Part model, mm, in its own coordinate system. A direction names the side the tool comes from. Give positions to 0.01 mm unless a question says otherwise; leave off trailing zeros. Order: outer loops, then holes, each group sorted by start corner. A loop starts at its lowest first (then second) coordinate and runs counter-clockwise, first axis right, second up. Notation, with made-up numbers: (23, -36) - (37, -36) arc R20 ccw to (37, -10) - close; hole circle Ø6 at (-17.75, -28.75). An arc over 180 degrees is marked (long way). Use a Markdown table: item, result. Add a question column.
from build123d import *

# Parameters (mm, degrees)
SALIENTE_EXTRUIR2_DEPTH    = 20
CORTAR_EXTRUIR1_DEPTH      = 109.18398602
CORTAR_EXTRUIR1_DEPTH_BACK = 109.18398602
CROQUIS3_R                 = 4
CROQUIS4_R                 = 2
CORTAR_EXTRUIR2_DEPTH      = 109.18398602


with BuildPart() as part:
    # Croquis1 → Saliente-Extruir2 (new body)
    with BuildSketch(Plane.XY):
        with BuildLine():
            Line((-57, 0), (-55.991070717, 0))
            ThreePointArc((-55.991070717, 0), (-55.290305828, -0.286607702), (-54.991230168, -0.982142857))
            ThreePointArc((-54.991230168, -0.982142857), (-41.300644472, -36.32157439), (-8, -54.415071442))
            Line((-8, -54.415071442), (-8, -56.435804238))
            Line((-8, -56.435804238), (-8, -71.312855839))
            Line((-8, -71.312855839), (8, -71.312855839))
            Line((8, -71.312855839), (8, -56.435804238))
            Line((8, -56.435804238), (8, -54.415071442))
            ThreePointArc((8, -54.415071442), (41.300644472, -36.32157439), (54.991230168, -0.982142857))
            ThreePointArc((54.991230168, -0.982142857), (55.290305828, -0.286607702), (55.991070717, 0))
            Line((55.991070717, 0), (57, 0))
            Line((57, 0), (76.5, 0))
            ThreePointArc((76.5, 0), (76.853553391, -0.146446609), (77, -0.5))
            Line((77, -0.5), (77, -1.5))
            ThreePointArc((77, -1.5), (76.853553391, -1.853553391), (76.5, -2))
            Line((76.5, -2), (57.92236183, -2))
            ThreePointArc((57.92236183, -2), (57.233785087, -2.274836523), (56.923700419, -2.948275862))
            ThreePointArc((56.923700419, -2.948275862), (42.736352788, -37.717425023), (10, -56.115951386))
            Line((10, -56.115951386), (10, -73.312855839))
            Line((10, -73.312855839), (-10, -73.312855839))
            Line((-10, -73.312855839), (-10, -56.115951386))
            ThreePointArc((-10, -56.115951386), (-42.736352788, -37.717425023), (-56.923700419, -2.948275862))
            ThreePointArc((-56.923700419, -2.948275862), (-57.233785087, -2.274836523), (-57.92236183, -2))
            Line((-57.92236183, -2), (-76.5, -2))
            ThreePointArc((-76.5, -2), (-76.853553391, -1.853553391), (-77, -1.5))
            Line((-77, -1.5), (-77, -0.5))
            ThreePointArc((-77, -0.5), (-76.853553391, -0.146446609), (-76.5, 0))
            Line((-76.5, 0), (-57, 0))
        make_face()
    extrude(amount=SALIENTE_EXTRUIR2_DEPTH)

    # Croquis3 → Cortar-Extruir1 (cut, two sides: drawn at the far end of the back side and taken through both)
    with BuildSketch(Plane.XZ.offset(73.312855839).offset(-CORTAR_EXTRUIR1_DEPTH_BACK)):
        with Locations(Location((0, 10, 0), (0, 0, 270))):
            Circle(CROQUIS3_R)
    extrude(amount=CORTAR_EXTRUIR1_DEPTH + CORTAR_EXTRUIR1_DEPTH_BACK, mode=Mode.SUBTRACT)

    # Croquis4 → Cortar-Extruir2 (cut, symmetric)
    with BuildSketch(Plane(origin=(0, 0, 0), x_dir=(1, 0, 0), z_dir=(0, 1, 0))):
        with Locations(Location((67, -10, 0), (0, 0, 270))):
            Circle(CROQUIS4_R)
    cortar_extruir2 = extrude(amount=CORTAR_EXTRUIR2_DEPTH, both=True, mode=Mode.SUBTRACT)

    # Simetría1: Cortar-Extruir2 across plane
    add(cortar_extruir2.mirror(Plane(origin=(0, 0, 0), x_dir=(0, 0, 1), z_dir=(1, 0, 0))), mode=Mode.SUBTRACT)


solid = part.part
1. Cut at A-A (x = -67). Write the cut outline in (y, z).
2. Drill centre lines: probe 1 along X at (y, z) = (-1.5, 10); probe 2 along X at (y, z) = (-72.5, 10); probe 3 along Z at (x, y) = (0, -72.65). Where is each one in solid material? Low to high. Write a range as [from, to].
3. Cut at D-D (x = -47). Write the cut outline in (y, z).
4. Mould opens along X. For faces 1 (the face through (43.1, -37.3, 9.9)), 2 (the face through (-66, 0, 12)), 3 (the face through (40.94, -36.73, 9.86)) say: released by +X, released by -X, zero draft, split by the parting line, or undercut.
5. Tool access for faces 4 (the face through (-4, -71.313, 8)), 5 (the face through (-10, -65, 10)), 6 (the face through (69.4, -2, 9.9)), 7 (the face through (69, -1, 10)): list every direction of +Z, -Z, +X, -X, +Y, -Y with a clear straight run to the whole face (end or side of a thin tool).
6. Cut at B-B (y = -66.5). Write the cut outline in (x, z).
7. Cut at C-C (z = 16). Write the cut outline in (x, y).
8. Pin check, flat tips, straight feed: P1, Ø9, axis at x = 0, z = 10, coming from the +Y side; P2, Ø8, axis at x = -17.5, z = 5.5, coming from the +Y side; P3, Ø8, axis at y = -26.5, z = 10, coming from the -X side; P4, Ø3, axis at x = 67, z = 10, coming from the -Y side. Stop position of each tip, or through.
Responses:
| question | item | result |
|---|---|---|
| 1 | outline | (-2, 0) - (0, 0) - (0, 8) - (-2, 8) - close; (-2, 12) - (0, 12) - (0, 20) - (-2, 20) - close |
| 2 | probe 1 | x = [-77, -69], [-65, -54.98], [54.98, 65], [69, 77] |
| 2 | probe 2 | x = [-10, -4], [4, 10] |
| 2 | probe 3 | z = [0, 6], [14, 20] |
| 3 | outline | (-32.25, 0) - (-28.57, 0) - (-28.57, 20) - (-32.25, 20) - close |
| 4 | face 1 | released by +X |
| 4 | face 2 | zero draft |
| 4 | face 3 | undercut |
| 5 | face 4 | +Z, -Z, +Y |
| 5 | face 5 | +Z, -Z, -X, -Y |
| 5 | face 6 | +Z, -Z, +X, -Y |
| 5 | face 7 | +Y, -Y |
| 6 | outline | (-10, 0) - (-8, 0) - (-8, 20) - (-10, 20) - close; (8, 0) - (10, 0) - (10, 20) - (8, 20) - close |
| 7 | outline | (-77, -1.5) arc R0.5 ccw to (-76.5, -2) - (-57.92, -2) arc R1 cw to (-56.92, -2.95) arc R57 ccw to (-10, -56.12) - (-10, -73.31) - (10, -73.31) - (10, -56.12) arc R57 ccw to (56.92, -2.95) arc R1 cw to (57.92, -2) - (76.5, -2) arc R0.5 ccw to (77, -1.5) - (77, -0.5) arc R0.5 ccw to (76.5, 0) - (55.99, 0) arc R1 ccw to (54.99, -0.98) arc R55 cw to (8, -54.42) - (8, -71.31) - (-8, -71.31) - (-8, -54.42) arc R55 cw to (-54.99, -0.98) arc R1 ccw to (-55.99, 0) - (-76.5, 0) arc R0.5 ccw to (-77, -0.5) - close |
| 8 | P1 | stops at y = -71.31 |
| 8 | P2 | stops at y = -50.62 |
| 8 | P3 | stops at x = -52.37 |
| 8 | P4 | passes through |
